Read the model definition and answer for the solid it produces. Units are mm, in the model's axes. A direction names the side the tool comes from. Coordinates: 2 decimals unless noted, no trailing zeros. Write each loop counter-clockwise with the first axis right and the second up, starting at its lowest first coordinate (ties: lowest second). Pieces come first, ordered by that corner, then holes. Notation, with made-up numbers: M 35.5,57.5 L 86.5,57.5 A20 cw 86.5,77.5 Z; hole C 73,-40 d1. An arc over 180 degrees is marked long. Use a Markdown table: item, result. Add a question column.
from build123d import *

# Parameters (mm, degrees)
SKIZZE1_R                       = 52
AUFSATZ_LINEAR_AUSTRAGEN1_DEPTH = 3
SKIZZE1_3_R                     = 55
SKIZZE1_3_R_2                   = 52
AUFSATZ_LINEAR_AUSTRAGEN2_DEPTH = 1.5
SCHNITT_LINEAR_AUSTRAGEN1_REACH = 5
SKIZZE3_R                       = 1.6
AUFSATZ_LINEAR_AUSTRAGEN3_DEPTH = 33
SCHNITT_LINEAR_AUSTRAGEN4_REACH = 99.7
SCHNITT_LINEAR_START            = -4
VERRUNDUNG1_R                   = 6
SCHNITT_LINEAR_AUSTRAGEN9_DEPTH = 6
VERRUNDUNG2_R                   = 6


with BuildPart() as part:
    # Skizze1 → Aufsatz-Linear austragen1 (new body)
    with BuildSketch(Plane.XY):
        Circle(SKIZZE1_R)
    extrude(amount=AUFSATZ_LINEAR_AUSTRAGEN1_DEPTH)

    # Skizze1_3 → Aufsatz-Linear austragen2 (add)
    with BuildSketch(Plane.XY):
        Circle(SKIZZE1_3_R)
        Circle(SKIZZE1_3_R_2, mode=Mode.SUBTRACT)
    extrude(amount=AUFSATZ_LINEAR_AUSTRAGEN2_DEPTH)

    # Skizze3 → Schnitt-Linear austragen1 (cut, up to next)
    with BuildSketch(Plane.XY.offset(3), mode=Mode.PRIVATE) as schnitt_linear_austragen1_sk1:
        with Locations((4.995000167, 4.995918163)):
            Circle(SKIZZE3_R)
    schnitt_linear_austragen1_tool1 = extrude(schnitt_linear_austragen1_sk1.sketch, amount=-SCHNITT_LINEAR_AUSTRAGEN1_REACH, mode=Mode.PRIVATE) & part.part
    add(schnitt_linear_austragen1_tool1.solids().sort_by_distance((4.995, 4.995918, 3))[0], mode=Mode.SUBTRACT)
    # Skizze3 → Schnitt-Linear austragen1 (cut, up to next)
    with BuildSketch(Plane.XY.offset(3), mode=Mode.PRIVATE) as schnitt_linear_austragen1_sk2:
        with Locations((4.995000167, 29.995918163)):
            Circle(SKIZZE3_R)
    schnitt_linear_austragen1_tool2 = extrude(schnitt_linear_austragen1_sk2.sketch, amount=-SCHNITT_LINEAR_AUSTRAGEN1_REACH, mode=Mode.PRIVATE) & part.part
    add(schnitt_linear_austragen1_tool2.solids().sort_by_distance((4.995, 29.995918, 3))[0], mode=Mode.SUBTRACT)
    # Skizze3 → Schnitt-Linear austragen1 (cut, up to next)
    with BuildSketch(Plane.XY.offset(3), mode=Mode.PRIVATE) as schnitt_linear_austragen1_sk3:
        with Locations((-30.004999833, 4.995918163)):
            Circle(SKIZZE3_R)
    schnitt_linear_austragen1_tool3 = extrude(schnitt_linear_austragen1_sk3.sketch, amount=-SCHNITT_LINEAR_AUSTRAGEN1_REACH, mode=Mode.PRIVATE) & part.part
    add(schnitt_linear_austragen1_tool3.solids().sort_by_distance((-30.005, 4.995918, 3))[0], mode=Mode.SUBTRACT)

    # Skizze2 → Aufsatz-Linear austragen3 (add)
    with BuildSketch(Plane.XY.offset(3)):
        Polygon((26, 21), (26, 16.2), (27.2, 16.2), (28.7, 16.2), (28.7, 15), (28.7, -24.5), (28.7, -25.7), (27.2, -25.7), (26, -25.7), (26, -26), (21, -26), (16.2, -26), (16.2, -27.2), (16.2, -28.7), (15, -28.7), (-24.5, -28.7), (-25.7, -28.7), (-25.7, -27.2), (-25.7, -26), (-30.5, -26), (-30.5, -33.3), (-24.5, -33.3), (-24.5, -38.7), (15, -38.7), (15, -33.3), (21, -33.3), (21, -30.5), (26, -30.5), (33.3, -30.5), (33.3, -24.5), (38.7, -24.5), (38.7, 15), (33.3, 15), (33.3, 21), align=None)
    extrude(amount=AUFSATZ_LINEAR_AUSTRAGEN3_DEPTH)

    # Skizze6 → Schnitt-Linear austragen4 (cut, up to next)
    with BuildSketch(Plane.XZ.offset(38.7).offset(SCHNITT_LINEAR_START), mode=Mode.PRIVATE) as schnitt_linear_austragen4_sk1:
        Polygon((-24.25, 3), (-23.25, 33), (13.75, 33), (14.75, 3), align=None)
    schnitt_linear_austragen4_tool1 = extrude(schnitt_linear_austragen4_sk1.sketch, amount=-SCHNITT_LINEAR_AUSTRAGEN4_REACH, mode=Mode.PRIVATE) & part.part
    add(schnitt_linear_austragen4_tool1.solids().sort_by_distance((-4.75, -34.7, 17.868421))[0], mode=Mode.SUBTRACT)

    # Verrundung1
    verrundung1_edges = [part.edges().sort_by_distance(p)[0] for p in [
        (-23.25, -31.7, 33),
        (13.75, -31.7, 33),
    ]]
    fillet(verrundung1_edges, radius=VERRUNDUNG1_R)

    # Skizze7 → Schnitt-Linear austragen9 (cut)
    with BuildSketch(Plane.ZY.offset(-28.7)):
        Polygon((33, -23.25), (33, 13.75), (3, 14.75), (3, -24.25), align=None)
    extrude(amount=-SCHNITT_LINEAR_AUSTRAGEN9_DEPTH, mode=Mode.SUBTRACT)

    # Verrundung2
    verrundung2_edges = [part.edges().sort_by_distance(p)[0] for p in [
        (31.7, -23.25, 33),
        (31.7, 13.75, 33),
    ]]
    fillet(verrundung2_edges, radius=VERRUNDUNG2_R)


solid = part.part
Item 1: Each of these flat-tipped pins is pushed along its axis until it touches: pin 1 (1.6 mm diameter, centred on y = -36.5, z = 21, fed in from +X); pin 2 (3 mm diameter, centred on x = 5, y = 5, fed in from +Z); pin 3 (3.5 mm diameter, centred on x = 30.5, z = 19, fed in from +Y); pin 4 (10 mm diameter, centred on x = -10, y = 31.5, fed in from -Z). Where does it stop, or does it pass through?
Item 2: Consider probe 1 along X at (y, z) = (-28, 22); probe 2 along Z at (x, y) = (-39.5, -33); probe 3 along Y at (x, z) = (17, 9.5). Determine where each line is inside the solid, lowest interval first.
Item 3: For faces 5 (the flat face through (-4, -34.7, 18)), 6 (the flat face through (28.7, -5, 34)), 7 (the cylindrical face through (31.74, -21.57, 31.36)), 8 (the flat face through (-28, -26, 19)), determine the directions among +Z, -Z, +X, -X, +Y, -Y from which every point of the face is accessible in a straight line to the end or side of a thin tool.
Item 4: Find section D-D on x = 31. Give the vertices of the cut face in (y, z).
Item 5: Determine the mould class of faces 1 (the flat face through (38.7, -5, 19)), 2 (the cylindrical face through (4.787, 31.582, 1.521)), 3 (the flat face through (30, 21, 19)), 4 (the cylindrical face through (-11.923, -53.692, 0.74)) for opening direction X: pulls with the +X half, pulls with the -X half, needs draft (parallel to the pull), parting line crosses it, or undercut.
Item 6: Find section B-B on x = 0. Give the vertices of the cut face in (y, z), then the cut area to 3 significant figures.
Item 7: Find section C-C on y = 0. Give the vertices of the cut face in (x, z).
Geometry says:
| question | item | result |
|---|---|---|
| 1 | pin 1 | stops at x = 15 |
| 1 | pin 2 | passes through |
| 1 | pin 3 | stops at y = 21 |
| 1 | pin 4 | stops at z = 0 |
| 2 | probe 1 | x = -30.5 to -25.7, 16.2 to 33.3 |
| 2 | probe 2 | z = 0 to 3 |
| 2 | probe 3 | y = -33.3 to -26 |
| 3 | face 5 | +Y |
| 3 | face 6 | +Z, -X |
| 3 | face 7 | -X |
| 3 | face 8 | +Z, -X, +Y |
| 4 | outline | M -45.43,0 L 45.43,0 L 45.43,1.5 L 41.75,1.5 L 41.75,3 L 21,3 L 21,36 L -30.5,36 L -30.5,3 L -41.75,3 L -41.75,1.5 L -45.43,1.5 Z; hole M -24.25,3 L 14.75,3 L 13.94,27.2 A6 ccw 7.95,33 L -17.45,33 A6 ccw -23.44,27.2 Z |
| 5 | face 1 | pulls with the +X half |
| 5 | face 2 | undercut |
| 5 | face 3 | needs draft |
| 5 | face 4 | parting line crosses it |
| 6 | outline | M -55,0 L 55,0 L 55,1.5 L 52,1.5 L 52,3 L -34.7,3 L -34.7,33 L -28.7,33 L -28.7,36 L -38.7,36 L -38.7,3 L -52,3 L -52,1.5 L -55,1.5 Z |
| 6 | area | 471 mm2 |
| 7 | outline | M -55,0 L 55,0 L 55,1.5 L 52,1.5 L 52,3 L 38.7,3 L 38.7,36 L 28.7,36 L 28.7,33 L 34.7,33 L 34.7,3 L -52,3 L -52,1.5 L -55,1.5 Z |
